Geometry check sheet. Reference: the model listing, model coordinates, mm. A direction names the side the tool comes from. Give positions to 0.01 mm unless a question says otherwise; leave off trailing zeros. Order: outer loops, then holes, each group sorted by start corner. A loop starts at its lowest first (then second) coordinate and runs counter-clockwise, first axis right, second up.
Autodesk Inventor part; units mm, degrees
ref_plane "YZ Plane" through (0, 0, 0) normal (1, 0, 0) x (0, 1, 0)
ref_plane "XZ Plane" through (0, 0, 0) normal (0, 1, 0) x (-1, 0, 0)
ref_plane "XY Plane" through (0, 0, 0) normal (0, 0, 1) x (1, 0, 0)
sketch "草图1" plane through (0, 0, 0) normal (0, 0, 1) x (1, 0, 0)
  circle A0 centre (-1.9411, 0.0503) radius 2.5
  line L0 (4.3454, -10.9196) -> (9.6453, -10.9355)
  circle A1 centre (-1.9411, 0.0503) radius 5.5
  line L1 (-1.9411, -10.9276) -> (10.9921, -10.9276)
  line L2 (10.9921, -10.9276) -> (10.9921, 5.5503)
  line L3 (10.9921, 5.5503) -> (-1.9411, 5.5503)
  line L4 (-1.9411, 5.5503) -> (-1.9411, -10.9276)
  point P0 (6.9953, -10.9276)
  point P1 (-1.9411, 5.5503)
  point P2 (-1.9411, -5.4497)
  dimension "d3" = 3
  dimension "d5" = 5
extrude "拉伸1" add sketch "草图1" along normal blind 3.5 contours A0 L4 A1 | A0 L4 A1 | L3 L2 L1 L4 A1
fillet "圆角1" radius 4 1 edges at (-1.9411, -5.4497, 1.75)
sketch "草图2" plane through (0, 0, 0) normal (0, 0, -1) x (-1, 0, 0)
  point P0 (0, 0)
sketch "草图3" plane through (0, 0, 0) normal (0, 0, -1) x (-1, 0, 0)
  circle A0 centre (1.9411, 0.0503) radius 2.5
  circle A1 centre (1.9411, 0.0503) radius 4
  point P0 (0, 0)
  dimension "d6" = 8
extrude "拉伸2" cut sketch "草图3" against normal blind 1 contours A0 | A1
sketch "草图4" plane through (-1.9411, -10.9276, 0) normal (0, -1, 0) x (1, 0, 0)
  ellipse E0 centre (8.9346, 1.75) end of major axis (8.9346, 0.85) minor radius 0.9
  point P0 (1.9411, 0)
extrude "拉伸3" cut sketch "草图4" against normal blind 3
fillet "圆角2" radius 1 2 edges at (10.9921, 5.5503, 1.75) (-1.9411, -10.9276, 1.75)
sketch "草图5" plane through (0, 0, 3.5) normal (0, 0, 1) x (1, 0, 0)
  line L0 (15.1126, -4.4497) -> (15.1126, -8.4497)
  line L1 (5.3617, -4.4497) -> (15.1126, -4.4497)
  line L2 (5.3617, -8.4497) -> (5.3617, -4.4497)
  line L3 (5.3617, -8.4497) -> (15.1126, -8.4497)
  line L4 (5.3617, -6.4497) -> (10.3955, -6.4497)
  circle A0 centre (7.8786, -6.4497) radius 0.8
  circle A1 centre (7.8786, -6.4497) radius 1
  point P0 (0, 0)
  dimension "d12" = 1.6
extrude "拉伸4" cut sketch "草图5" against normal blind 5.5 contours A0 L4 | L4 A0
sketch "草图6" plane through (0, 0, 3.5) normal (0, 0, 1) x (1, 0, 0)
  circle A0 centre (7.8786, -2.4497) radius 0.8
  circle A1 centre (7.8786, -6.4497) radius 0.8
  line L0 (7.8786, -6.4497) -> (7.8786, 5.5503)
  line L1 (9.9921, 5.5503) -> (-1.9411, 5.5503)
  point P0 (0, 0)
  dimension "d17" = 1.6
extrude "拉伸5" cut sketch "草图6" against normal blind 10 contours A0 L0 | L0 A0
sketch "草图7" plane through (10.9921, -10.9276, 0) normal (0, -1, 0) x (1, 0, 0)
  ellipse E0 centre (-3.9986, 1.75) end of major axis (-3.9986, 0.85) minor radius 0.9
  circle A0 centre (-3.9986, 1.75) radius 0.8
  point P0 (-10.9921, 0)
  dimension "d18" = 1.6
extrude "拉伸6" add sketch "草图7" against normal up to surface (3 mm away)
properties part number "针头装配体"
Item 1: Scan lines: L1, parallel to Y at x = 7.25, z = 2; L2, parallel to X at y = 1, z = 1.6; L3, parallel to X at y = 3.5, z = 0.8. Record each from-to range of solid material in increasing order.
Reported:
L1: y = -7.93 to -6.94, -5.95 to -2.94, -1.95 to 5.55
L2: x = -7.36 to -4.25, 0.37 to 10.99
L3: x = -6.22 to -3.97, 0.08 to 10.99
Item 2: Sectioned sample at B-B (z = 2.3). Enter the section's corners in (x, y).
Reported:
outline: (-4.26, -4.94) arc R4 cw to (-1.94, -8.57) - (-1.94, -9.93) arc R1 ccw to (-0.94, -10.93) - (6.41, -10.93) - (6.41, -7.93) - (7.57, -7.93) - (7.57, -10.93) - (10.99, -10.93) - (10.99, 4.55) arc R1 ccw to (9.99, 5.55) - (-1.94, 5.55) arc R5.5 ccw to start; hole circle Ø5 at (-1.94, 0.05); hole circle Ø1.6 at (7.88, -6.45); hole circle Ø1.6 at (7.88, -2.45)
Item 3: Draft check along Z on faces 1 (the cylindrical face through (0.443, -0.701, 2.232)), 2 (the flat face through (4, -3, 0)), 3 (the cylindrical face through (6.194, -9.449, 1.785)), 4 (the flat face through (7, -7.928, 2)). Enter one of: released by +Z, released by -Z, zero draft, split by the parting line, or undercut.
Reported:
face 1: zero draft
face 2: released by -Z
face 3: undercut
face 4: undercut
Item 4: Gauge pin test, flat ends, axial feed: pin 1 (1.5 mm diameter, centred on x = -5.5, z = 2, fed in from +Y); pin 2 (3 mm diameter, centred on x = -1.94, y = 0.05, fed in from +Z); pin 3 (5 mm diameter, centred on x = 1, y = -3, fed in from -Z); pin 4 (1.3 mm diameter, centred on x = 6.99, z = 1.75, fed in from -Y). Record the tip position at first contact, or that the pin passes through.
Reported:
pin 1: stops at y = 4.78
pin 2: passes through
pin 3: stops at z = 0
pin 4: stops at y = -7.93
Item 5: Sectioned sample at C-C (x = -3). Enter the section's corners in (y, z), and give its area (3 significant figures).
Reported:
outline: (-5.86, 0) - (-3.81, 0) - (-3.81, 1) - (-2.21, 1) - (-2.21, 3.5) - (-5.86, 3.5) - close; (2.31, 1) - (3.91, 1) - (3.91, 0) - (5.45, 0) - (5.45, 3.5) - (2.31, 3.5) - close
area: 20.5 mm2
Item 6: Sectioned sample at D-D (z = 0.55). Enter the section's corners in (x, y), and give its area (3 significant figures).
Reported:
outline: (-4.26, -4.94) arc R4 cw to (-1.94, -8.57) - (-1.94, -9.93) arc R1 ccw to (-0.94, -10.93) - (10.99, -10.93) - (10.99, 4.55) arc R1 ccw to (9.99, 5.55) - (-1.94, 5.55) arc R5.5 ccw to start; hole circle Ø8 at (-1.94, 0.05); hole circle Ø1.6 at (7.88, -6.45); hole circle Ø1.6 at (7.88, -2.45)
area: 207 mm2
Item 7: Set-up check for faces 5 (the flat face through (-1.941, -9, 2)), 6 (the flat face through (4, -3, 3.5)), 7 (the flat face through (0, -2, 1)): record each of +Z, -Z, +X, -X, +Y, -Y from which the full face is reachable in a straight line by a thin tool's end or side.
Reported:
face 5: +Z, -Z, -X, -Y
face 6: +Z, +X, -X, +Y, -Y
face 7: -Z
Item 8: Sectioned sample at A-A (y = -1.25). Enter the section's corners in (x, z).
Reported:
outline: (-7.29, 0) - (-5.72, 0) - (-5.72, 1) - (-4.08, 1) - (-4.08, 3.5) - (-7.29, 3.5) - close; (0.19, 1) - (1.84, 1) - (1.84, 0) - (10.99, 0) - (10.99, 3.5) - (0.19, 3.5) - close
